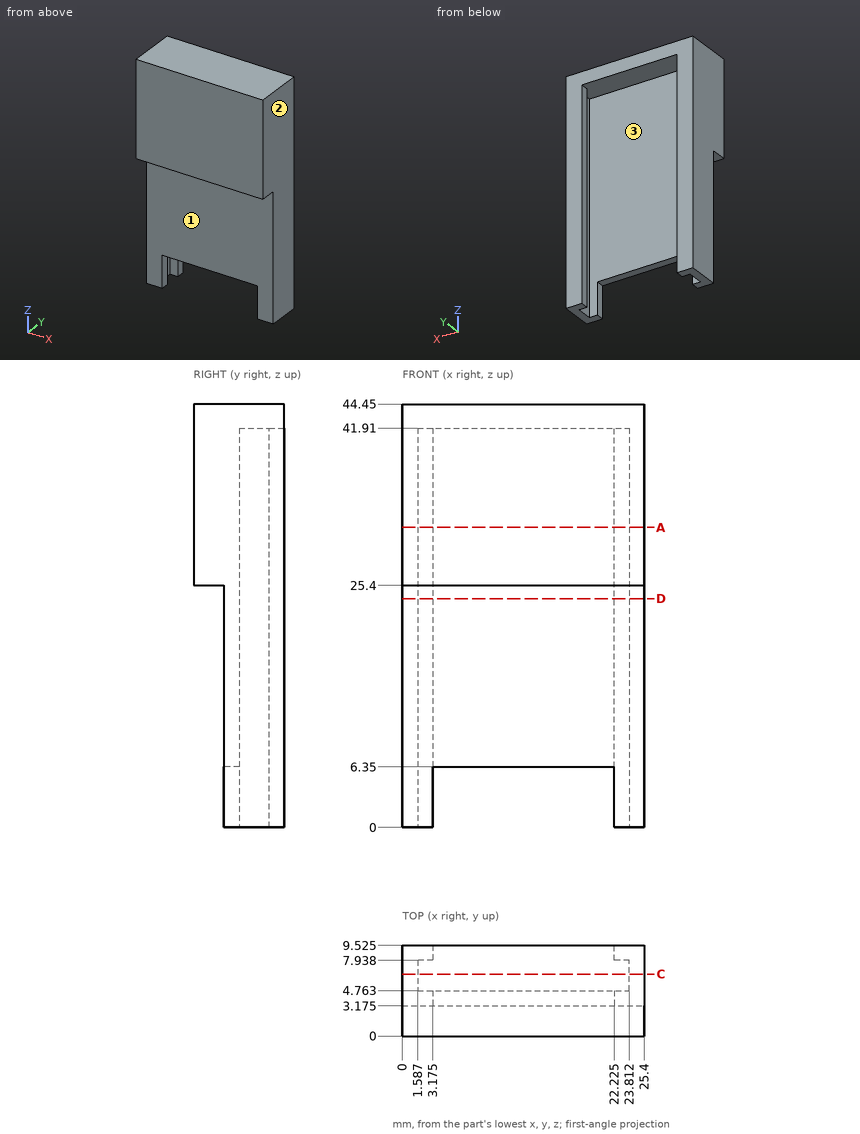
Part print with two shaded views. Sizes in mm from the minimum x, y, z corner. Round coordinates to 2 decimals unless told otherwise and drop trailing zeros. Order: outer loops, then holes, each group sorted by start corner. A loop starts at its lowest first (then second) coordinate and runs counter-clockwise, first axis right, second up. Notation, with made-up numbers: (36, 50) -> (90, 50) arc R20 ccw to (90, 59) -> close; hole circle Ø10 at (45, -23.75). An arc over 180 degrees is marked (long way). Write each question's results on one line, items separated by ' | '.
1. Flat gauge pins, fed straight in: P1, Ø0.5, axis at y = 3.5, z = 3, coming from the -X side; P2, Ø7.5, axis at x = 9.5, z = 11.5, coming from the -Y side (1 decimal); P3, Ø4, axis at x = 8.5, y = 2, coming from the -Z side; P4, Ø2, axis at y = 2, z = 23, coming from the +X side. Where does each tip first touch, or does it go through?
Findings below:
P1: stops at x = 0 | P2: stops at y = 3.2 | P3: stops at z = 6.35 | P4: passes through
2. Pull direction Y, two halves, no side cores. Call the marked faces 1, 2 and 3: pulls with the +Y half, pulls with the -Y half, needs draft (parallel to the pull), parting line crosses it, or undercut.
Findings below:
face 1: pulls with the -Y half | face 2: needs draft | face 3: undercut
3. Cut at C-C (y = 6.5). Give the cut face in (x, z).
Findings below:
outline: (0, 0) -> (1.59, 0) -> (1.59, 41.91) -> (23.81, 41.91) -> (23.81, 0) -> (25.4, 0) -> (25.4, 44.45) -> (0, 44.45) -> close
4. Wall check: line 1 along X through (y, z) = (9.25, 41) (1 decimal); line 2 along X through (y, z) = (7.25, 24); line 3 along Y through (x, z) = (2.25, 22.5) (1 decimal). Give the ranges that are in metal, low to high. Write a range as [from, to].
Findings below:
line 1: x = [0, 3.2], [22.2, 25.4] | line 2: x = [0, 1.59], [23.81, 25.4] | line 3: y = [3.2, 4.8], [7.9, 9.5]
5. Cut at A-A (z = 31.5). Give the cut face in (x, y) (1 decimal).
Findings below:
outline: (0, 0) -> (25.4, 0) -> (25.4, 9.5) -> (22.2, 9.5) -> (22.2, 7.9) -> (23.8, 7.9) -> (23.8, 4.8) -> (1.6, 4.8) -> (1.6, 7.9) -> (3.2, 7.9) -> (3.2, 9.5) -> (0, 9.5) -> close
6. Cut at D-D (z = 24). Give the cut face in (x, y) (1 decimal).
Findings below:
outline: (0, 3.2) -> (25.4, 3.2) -> (25.4, 9.5) -> (22.2, 9.5) -> (22.2, 7.9) -> (23.8, 7.9) -> (23.8, 4.8) -> (1.6, 4.8) -> (1.6, 7.9) -> (3.2, 7.9) -> (3.2, 9.5) -> (0, 9.5) -> close
